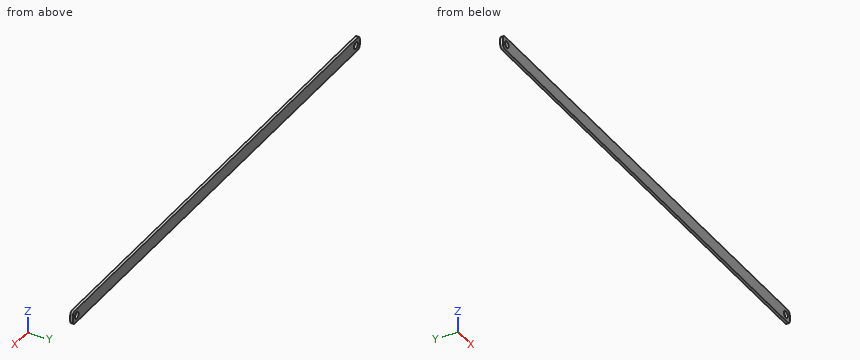
```python
from build123d import *

# Parameters (mm, degrees)
SKETCH1_R           = 2.5
BOSS_EXTRUDE2_DEPTH = 2
FLEX1_OUTLINE_R     = 2.5
FLEX1_DEPTH         = 2


# Read off the part's stored shape, not the designer's step: Flex1
with BuildPart() as part:
    # Sketch1 → Boss-Extrude2 (new body)
    with BuildSketch(Plane(origin=(0, 0, 0), x_dir=(1, 0, 0), z_dir=(0, 1, 0))):
        with BuildLine():
            Line((2.5, 0), (47.5, 0))
            ThreePointArc((47.5, 0), (49.267766953, 0.732233047), (50, 2.5))
            Line((50, 2.5), (50, 7.5))
            ThreePointArc((50, 7.5), (49.267766953, 9.267766953), (47.5, 10))
            Line((47.5, 10), (2.5, 10))
            ThreePointArc((2.5, 10), (0.732233047, 9.267766953), (0, 7.5))
            Line((0, 7.5), (0, 2.5))
            ThreePointArc((0, 2.5), (0.732233047, 0.732233047), (2.5, 0))
        make_face()
        with Locations(Location((5, 5, 0), (0, 0, 270))):
            Circle(SKETCH1_R, mode=Mode.SUBTRACT)
        with Locations(Location((45, 5, 0), (0, 0, 270))):
            Circle(SKETCH1_R, mode=Mode.SUBTRACT)
    extrude(amount=BOSS_EXTRUDE2_DEPTH)

    # Flex1 outline → Flex1 (add)
    # profile 1 of 4: a face of its own
    with BuildSketch(Plane(origin=(0, 0, 0), x_dir=(1, 0, 0), z_dir=(0, 1, 0))):
        with BuildLine():
            Line((2.5, 10), (-152.172258813, 10))
            ThreePointArc((-152.172258813, 10), (-153.940025766, 9.267766953), (-154.672258813, 7.5))
            Line((-154.672258813, 7.5), (-154.672258813, 2.5))
            ThreePointArc((-154.672258813, 2.5), (-153.940025766, 0.732233047), (-152.172258813, 0))
            Line((-152.172258813, 0), (2.5, 0))
            ThreePointArc((2.5, 0), (0.732233047, 0.732233047), (0, 2.5))
            Line((0, 2.5), (0, 7.5))
            ThreePointArc((0, 7.5), (0.732233047, 9.267766953), (2.5, 10))
        make_face()
        with Locations((-149.672258813, 5)):
            Circle(FLEX1_OUTLINE_R, mode=Mode.SUBTRACT)
    # profile 2 of 4: a face of its own
    with BuildSketch(Plane(origin=(0, 0, 0), x_dir=(1, 0, 0), z_dir=(0, 1, 0))):
        with BuildLine():
            Line((209.827741187, 10), (47.5, 10))
            ThreePointArc((47.5, 10), (49.267766953, 9.267766953), (50, 7.5))
            Line((50, 7.5), (50, 2.5))
            ThreePointArc((50, 2.5), (49.267766953, 0.732233047), (47.5, 0))
            Line((47.5, 0), (209.827741187, 0))
            ThreePointArc((209.827741187, 0), (211.59550814, 0.732233047), (212.327741187, 2.5))
            Line((212.327741187, 2.5), (212.327741187, 7.5))
            ThreePointArc((212.327741187, 7.5), (211.59550814, 9.267766953), (209.827741187, 10))
        make_face()
        with Locations((207.327741187, 5)):
            Circle(FLEX1_OUTLINE_R, mode=Mode.SUBTRACT)
    # profile 3 of 4: a face of its own
    with BuildSketch(Plane(origin=(0, 0, 0), x_dir=(1, 0, 0), z_dir=(0, 1, 0))):
        with Locations((5, 5)):
            Circle(FLEX1_OUTLINE_R)
    # profile 4 of 4: a face of its own
    with BuildSketch(Plane(origin=(0, 0, 0), x_dir=(1, 0, 0), z_dir=(0, 1, 0))):
        with Locations((45, 5)):
            Circle(FLEX1_OUTLINE_R)
    extrude(amount=FLEX1_DEPTH)


solid = part.part
```
Work out the finished part from the listing and answer in its coordinate system (mm). Round coordinates to 2 decimals unless told otherwise and drop trailing zeros. Write each loop counter-clockwise with the first axis right and the second up, starting at its lowest first coordinate (ties: lowest second). Pieces come first, ordered by that corner, then holes. Notation, with made-up numbers: (-24.75, 23.5) - (6.25, 23.5) arc R14 ccw to (6.25, 41.5) - close; hole circle Ø4 at (83, 66). An arc over 180 degrees is marked (long way). Return JSON: item names as keys, results as strings. Group by question number.
Q1. The part is cut by section A-A on z = -5. Write down the section's boundary in (x, y).
Q2. This flat-tipped pin is pushed along its axis until it touches: pin 1 Ø1 at (y, z) = (1.5, -9) entering from -X. Where does it stop, or does it pass through?
Q3. Find the intervals of material crossed by L1, parallel to X at y = 0.7, z = -5; L2, parallel to X at y = 1.5, z = -6.5; L3, parallel to X at y = 0.95, z = -8, in increasing order.
Solved:
{
 "1": {"outline": "(-154.67, 0) - (-152.17, 0) - (-152.17, 2) - (-154.67, 2) - close; (-147.17, 0) - (204.83, 0) - (204.83, 2) - (-147.17, 2) - close; (209.83, 0) - (212.33, 0) - (212.33, 2) - (209.83, 2) - close"},
 "2": {"pin 1": "x = -154.46"},
 "3": {"L1": "-154.67 to -152.17, -147.17 to 204.83, 209.83 to 212.33", "L2": "-154.67 to -151.67, -147.67 to 205.33, 209.33 to 212.33", "L3": "-154.62 to 212.28"}
}
